```python
from build123d import *

# Parameters (mm, degrees)
EXTRUDE_1_DEPTH     = 30
SKETCH_2_R          = 4.025
EXTRUDE_2_DEPTH     = 10.5
CHAMFER_1_SIZE      = 0.6
CUT_EXTRUDE_1_DEPTH = 8
CHAMFER_2_SIZE      = 1.5


with BuildPart() as part:
    # 草图1 → 凸台-拉伸1 (new body)
    with BuildSketch(Plane.XY):
        Polygon((5.773502692, 0), (2.886751346, 5), (-2.886751346, 5), (-5.773502692, 0), (-2.886751346, -5), (2.886751346, -5), align=None)
    extrude(amount=EXTRUDE_1_DEPTH)

    # 草图2 → 凸台-拉伸2 (add)
    with BuildSketch(Plane.XY.offset(30)):
        with Locations(Location((0, 0, 0), (0, 0, 180))):
            Circle(SKETCH_2_R)
    extrude(amount=EXTRUDE_2_DEPTH)

    # 倒角1
    chamfer_1_edges = [part.edges().sort_by_distance(p)[0] for p in [
        (4.025, 0, 40.5),
    ]]
    chamfer(chamfer_1_edges, length=CHAMFER_1_SIZE)

    # 草图3 → 切除-拉伸1 (cut)
    with BuildSketch(Plane.XY.offset(40.5)):
        with BuildLine():
            Line((-1.140175425, 1.05), (1.140175425, 1.05))
            ThreePointArc((1.140175425, 1.05), (0, -1.55), (-1.140175425, 1.05))
        make_face()
    extrude(amount=-CUT_EXTRUDE_1_DEPTH, mode=Mode.SUBTRACT)

    # 倒角2
    # the kernel refuses this chamfer: 1.5 mm, written as the material it takes off along each edge
    with BuildSketch(Plane(origin=(6.744275828, 5, 30), x_dir=(3.229355886475551e-15, -0.9996219169112968, 0.027495876610586775), z_dir=(-1, 0, 0))) as chamfer_2_piece_1_section:
        Polygon((CHAMFER_2_SIZE * 0.999621916911, -CHAMFER_2_SIZE * 0.0274958766106), (-CHAMFER_2_SIZE * 0.0274958766106, -CHAMFER_2_SIZE * 0.999621916911), (0, 0), align=None)
    chamfer_2_piece_1 = extrude(amount=13.488551656, mode=Mode.PRIVATE)
    chamfer_2_piece_1 = chamfer_2_piece_1 - Plane(origin=(0, 0, 29.496283425), x_dir=(-1, 0, 0), z_dir=(0, 0, -1)) * Cylinder(4.025, 33, mode=Mode.PRIVATE)
    add(chamfer_2_piece_1, mode=Mode.SUBTRACT)
    with BuildSketch(Plane(origin=(-0.957989105, 8.340714197, 30), x_dir=(0.865697974224883, -0.49981095845564333, 0.02749587661058677), z_dir=(-0.49999999999999506, -0.8660254037844416, 0))) as chamfer_2_piece_2_section:
        Polygon((CHAMFER_2_SIZE * 0.999621916911, -CHAMFER_2_SIZE * 0.0274958766106), (-CHAMFER_2_SIZE * 0.0274958766106, -CHAMFER_2_SIZE * 0.999621916911), (0, 0), align=None)
    chamfer_2_piece_2 = extrude(amount=13.488551656, mode=Mode.PRIVATE)
    chamfer_2_piece_2 = chamfer_2_piece_2 - Plane(origin=(0, 0, 29.496283425), x_dir=(-1, 0, 0), z_dir=(0, 0, -1)) * Cylinder(4.025, 33, mode=Mode.PRIVATE)
    add(chamfer_2_piece_2, mode=Mode.SUBTRACT)
    with BuildSketch(Plane(origin=(-7.702264933, 3.340714197, 30), x_dir=(0.8656979742248763, 0.49981095845565543, 0.02749587661058678), z_dir=(0.5000000000000071, -0.8660254037844346, 0))) as chamfer_2_piece_3_section:
        Polygon((CHAMFER_2_SIZE * 0.999621916911, -CHAMFER_2_SIZE * 0.0274958766106), (-CHAMFER_2_SIZE * 0.0274958766106, -CHAMFER_2_SIZE * 0.999621916911), (0, 0), align=None)
    chamfer_2_piece_3 = extrude(amount=13.488551656, mode=Mode.PRIVATE)
    chamfer_2_piece_3 = chamfer_2_piece_3 - Plane(origin=(0, 0, 29.496283426), x_dir=(-1, 0, 0), z_dir=(0, 0, -1)) * Cylinder(4.025, 33, mode=Mode.PRIVATE)
    add(chamfer_2_piece_3, mode=Mode.SUBTRACT)
    with BuildSketch(Plane(origin=(-6.744275828, -5, 30), x_dir=(-1.061074076984824e-14, 0.9996219169112968, 0.027495876610586775), z_dir=(1, 0, 0))) as chamfer_2_piece_4_section:
        Polygon((CHAMFER_2_SIZE * 0.999621916911, -CHAMFER_2_SIZE * 0.0274958766106), (-CHAMFER_2_SIZE * 0.0274958766106, -CHAMFER_2_SIZE * 0.999621916911), (0, 0), align=None)
    chamfer_2_piece_4 = extrude(amount=13.488551656, mode=Mode.PRIVATE)
    chamfer_2_piece_4 = chamfer_2_piece_4 - Plane(origin=(0, 0, 29.496283425), x_dir=(-1, 0, 0), z_dir=(0, 0, -1)) * Cylinder(4.025, 33, mode=Mode.PRIVATE)
    add(chamfer_2_piece_4, mode=Mode.SUBTRACT)
    with BuildSketch(Plane(origin=(0.957989105, -8.340714197, 30), x_dir=(-0.865697974224883, 0.49981095845564333, 0.02749587661058677), z_dir=(0.49999999999999506, 0.8660254037844416, 0))) as chamfer_2_piece_5_section:
        Polygon((CHAMFER_2_SIZE * 0.999621916911, -CHAMFER_2_SIZE * 0.0274958766106), (-CHAMFER_2_SIZE * 0.0274958766106, -CHAMFER_2_SIZE * 0.999621916911), (0, 0), align=None)
    chamfer_2_piece_5 = extrude(amount=13.488551656, mode=Mode.PRIVATE)
    chamfer_2_piece_5 = chamfer_2_piece_5 - Plane(origin=(0, 0, 29.496283425), x_dir=(-1, 0, 0), z_dir=(0, 0, -1)) * Cylinder(4.025, 33, mode=Mode.PRIVATE)
    add(chamfer_2_piece_5, mode=Mode.SUBTRACT)
    with BuildSketch(Plane(origin=(7.702264933, -3.340714197, 30), x_dir=(-0.8656979742248796, -0.4998109584556494, 0.02749587661058677), z_dir=(-0.5000000000000011, 0.866025403784438, 0))) as chamfer_2_piece_6_section:
        Polygon((CHAMFER_2_SIZE * 0.999621916911, -CHAMFER_2_SIZE * 0.0274958766106), (-CHAMFER_2_SIZE * 0.0274958766106, -CHAMFER_2_SIZE * 0.999621916911), (0, 0), align=None)
    chamfer_2_piece_6 = extrude(amount=13.488551656, mode=Mode.PRIVATE)
    chamfer_2_piece_6 = chamfer_2_piece_6 - Plane(origin=(0, 0, 29.496283425), x_dir=(-1, 0, 0), z_dir=(0, 0, -1)) * Cylinder(4.025, 33, mode=Mode.PRIVATE)
    add(chamfer_2_piece_6, mode=Mode.SUBTRACT)

    # 草图4 → 切除-旋转4 (revolve, cut)
    with BuildSketch(Plane(origin=(0, 0, 0), x_dir=(0, 0, -1), z_dir=(1, 0, 0)), mode=Mode.PRIVATE) as cut_revolve_4_sk:
        Polygon((-6.5, 6.5), (0.5, 6.5), (-3, 3), align=None)
    revolve(cut_revolve_4_sk.sketch.rotate(Axis((0, 0, -6.39558723), (0, 0, 1)), 89.591845794), axis=Axis((0, 0, -6.39558723), (0, 0, 1)), mode=Mode.SUBTRACT)


solid = part.part
```
The model under review builds one solid part; all positions refer to its coordinate system, in mm. A direction names the side the tool comes from. Round coordinates to 2 decimals unless told otherwise and drop trailing zeros. Order: outer loops, then holes, each group sorted by start corner. A loop starts at its lowest first (then second) coordinate and runs counter-clockwise, first axis right, second up.
(1) Take a section at C-C, the plane z = 3.5. State the section outline as (x, y) points.
Working result:
outline: circle Ø7 at (0, 0)
(2) Take a section at A-A, the plane x = 0. State the section outline as (y, z) points (3 decimals).
Working result:
outline: (-5, 0) - (5, 0) - (5, 1) - (3, 3) - (5, 5) - (5, 28.5) - (4.025, 29.475) - (4.025, 39.9) - (3.425, 40.5) - (1.05, 40.5) - (1.05, 32.5) - (-1.55, 32.5) - (-1.55, 40.5) - (-3.425, 40.5) - (-4.025, 39.9) - (-4.025, 29.475) - (-5, 28.5) - (-5, 5) - (-3, 3) - (-5, 1) - close
(3) For P1, Ø1.5, axis at y = -1, z = 17.5, coming from the -X side; P2, Ø1.8, axis at x = 0, z = 35, coming from the -Y side (3 decimals); P3, Ø2, axis at y = -2.5, z = 6, coming from the -X side, all flat-tipped, find the tip position at first contact; note any pin that passes through.
Working result:
P1: stops at x = -5.63
P2: stops at y = -4.025
P3: stops at x = -4.91
(4) Wall thickness on L1, parallel to Y at x = 0, z = 38.75 (3 decimals); L2, parallel to Z at x = -1, y = -3.5; L3, parallel to X at y = -0.25, z = 37.5: over which ranges is each line inside the solid? List them lowest first.
Working result:
L1: y = -4.025 to -1.55, 1.05 to 4.025
L2: z = 0 to 2.36, 3.64 to 40.28
L3: x = -4.02 to -1.53, 1.53 to 4.02
(5) Mouldability with a two-part tool opening along Z and no side actions: class faces 1 (the face through (0, 0, 32.5)), 2 (the face through (0, 5, 0.4)), 3 (the face through (0.701, 3.055, 2.865)) as released by +Z, released by -Z, zero draft, split by the parting line, or undercut.
Working result:
face 1: released by +Z
face 2: zero draft
face 3: undercut
(6) Take a section at B-B, the plane z = 9. State the section outline as (x, y) points.
Working result:
outline: (-5.77, 0) - (-2.89, -5) - (2.89, -5) - (5.77, 0) - (2.89, 5) - (-2.89, 5) - close
(7) Tool access review of faces 4 (the face through (-4.31, 2.535, 0.382)), 5 (the face through (0.05, -1.55, 36.56)), 6 (the face through (-1.444, 2.826, 3.173)): name each direction out of +Z, -Z, +X, -X, +Y, -Y from which nothing blocks a thin tool from reaching the whole face with its end or side.
Working result:
face 4: +Z, -Z, -X, +Y
face 5: +Z
face 6: none
